```python
from build123d import *

# Parameters (mm, degrees)
SKETCH2_W           = 54
SKETCH2_H           = 6.2
BOSS_EXTRUDE2_DEPTH = 12.5
SKETCH3_R           = 2.8
CUT_EXTRUDE1_DEPTH  = 6.2
CUT_EXTRUDE2_DEPTH  = 1.9
SKETCH6_W           = 8.1
SKETCH6_H           = 4
CUT_EXTRUDE3_DEPTH  = 8.65741
SKETCH7_W           = 3
SKETCH7_H           = 25
BOSS_EXTRUDE3_DEPTH = 7.9
CUT_EXTRUDE4_DEPTH  = 2
SKETCH9_R           = 0.7
CUT_EXTRUDE5_DEPTH  = 2
SKETCH13_W          = 54
SKETCH13_H          = 2.82
CUT_EXTRUDE6_DEPTH  = 33.925066439
SKETCH18_W          = 3
SKETCH18_H          = 2.82
CUT_EXTRUDE9_DEPTH  = 10
SKETCH19_W          = 0.539072716
SKETCH19_H          = 14.1
CUT_EXTRUDE11_DEPTH = 57.508848865
CUT_EXTRUDE13_DEPTH = 2.5
CUT_EXTRUDE15_START = -2
SKETCH23_R          = 1.6
CUT_EXTRUDE15_DEPTH = 7
CUT_EXTRUDE16_DEPTH = 1.2
SKETCH26_W          = 5.64
SKETCH26_H          = 2.8
CUT_EXTRUDE17_DEPTH = 2.3
SKETCH29_W          = 9
SKETCH29_H          = 3
BOSS_EXTRUDE5_DEPTH = 7.9
SKETCH34_W          = 9
SKETCH34_H          = 7.9
BOSS_EXTRUDE6_DEPTH = 7.5
CUT_EXTRUDE19_DEPTH = 9
CUT_EXTRUDE20_DEPTH = 2.5
SKETCH31_R          = 1.5
CUT_EXTRUDE18_DEPTH = 37.30881069


with BuildPart() as part:
    # Sketch2 → Boss-Extrude2 (new, symmetric)
    with BuildSketch(Plane(origin=(10.528308017, 2.71655886, 0), x_dir=(1, 0, 0), z_dir=(0, 0, 1))):
        with Locations((-10.528308017, -2.71655886)):
            Rectangle(SKETCH2_W, SKETCH2_H)
    extrude(amount=BOSS_EXTRUDE2_DEPTH, both=True)

    # Sketch3 → Cut-Extrude1 (cut)
    with BuildSketch(Plane.XZ.offset(3.1)):
        with Locations((-12.165967216, -142.374755929)):
            Circle(SKETCH3_R)
    extrude(amount=-CUT_EXTRUDE1_DEPTH, mode=Mode.SUBTRACT)

    # Sketch4 → Cut-Extrude2 (cut, symmetric)
    with BuildSketch(Plane(origin=(0, 0, 0), x_dir=(1, 0, 0), z_dir=(0, 1, 0))):
        Polygon((-10.635076842, 0.660738766), (-14.535076842, 2.912404816), (-18.435076842, 0.660738766), (-18.435076842, -3.842593333), (-14.535076842, -6.094259383), (-10.635076842, -3.842593333), align=None)
    extrude(amount=CUT_EXTRUDE2_DEPTH, both=True, mode=Mode.SUBTRACT)

    # Sketch6 → Cut-Extrude3 (cut)
    with BuildSketch(Plane.XY.offset(12.5)):
        with Locations((-14.535076842, 0)):
            Rectangle(SKETCH6_W, SKETCH6_H)
    extrude(amount=-CUT_EXTRUDE3_DEPTH, mode=Mode.SUBTRACT)

    # Sketch7 → Boss-Extrude3 (add)
    with BuildSketch(Plane.XZ.offset(3.1)):
        with Locations((-25.5, 0)):
            Rectangle(SKETCH7_W, SKETCH7_H)
    boss_extrude3 = extrude(amount=BOSS_EXTRUDE3_DEPTH)

    # Sketch8 → Cut-Extrude4 (cut)
    with BuildSketch(Plane.ZY.offset(27)):
        with BuildLine():
            Line((-1.559072716, -7.9), (-1.559072716, -11))
            Line((-1.559072716, -11), (4.740927284, -11))
            Line((4.740927284, -11), (4.740927284, -7.9))
            ThreePointArc((4.740927284, -7.9), (1.590927284, -4.75), (-1.559072716, -7.9))
        make_face()
    cut_extrude4 = extrude(amount=-CUT_EXTRUDE4_DEPTH, mode=Mode.SUBTRACT)

    # Sketch9 → Cut-Extrude5 (cut)
    with BuildSketch(Plane(origin=(-24, 0, 0), x_dir=(0, 0, -1), z_dir=(1, 0, 0))):
        with Locations((142.374755929, -8.1)):
            Circle(SKETCH9_R)
    cut_extrude5 = extrude(amount=-CUT_EXTRUDE5_DEPTH, mode=Mode.SUBTRACT)

    # Sketch13 → Cut-Extrude6 (cut, through all)
    with BuildSketch(Plane(origin=(0, 3.1, 0), x_dir=(1, 0, 0), z_dir=(0, 1, 0))):
        with Locations((0, 11.09)):
            Rectangle(SKETCH13_W, SKETCH13_H)
    extrude(amount=-CUT_EXTRUDE6_DEPTH, mode=Mode.SUBTRACT)

    # Mirror1: Boss-Extrude3, Cut-Extrude4, Cut-Extrude5 across plane
    add(boss_extrude3.mirror(Plane.ZY.offset(14.535076842)))
    add(cut_extrude4.mirror(Plane.ZY.offset(14.535076842)), mode=Mode.SUBTRACT)
    add(cut_extrude5.mirror(Plane.ZY.offset(14.535076842)), mode=Mode.SUBTRACT)

    # Sketch18 → Cut-Extrude9 (cut)
    with BuildSketch(Plane(origin=(0, -3.1, 0), x_dir=(1, 0, 0), z_dir=(0, 1, 0))):
        with Locations((-3.570153685, 11.09)):
            Rectangle(SKETCH18_W, SKETCH18_H)
    extrude(amount=-CUT_EXTRUDE9_DEPTH, mode=Mode.SUBTRACT)

    # Sketch19 → Cut-Extrude11 (cut, through all)
    with BuildSketch(Plane.ZY.offset(27)):
        with Locations((12.230463642, -3.95)):
            Rectangle(SKETCH19_W, SKETCH19_H)
    extrude(amount=-CUT_EXTRUDE11_DEPTH, mode=Mode.SUBTRACT)

    # Sketch22 → Cut-Extrude13 (cut)
    with BuildSketch(Plane.XZ.offset(3.1)):
        Polygon((15, 10.472778345), (12.15, 8.827330078), (12.15, 5.536433544), (15, 3.890985277), (17.85, 5.536433544), (17.85, 8.827330078), align=None)
        Polygon((15, -2.584684642), (12.15, -4.230132909), (12.15, -7.521029443), (15, -9.16647771), (17.85, -7.521029443), (17.85, -4.230132909), align=None)
    extrude(amount=-CUT_EXTRUDE13_DEPTH, mode=Mode.SUBTRACT)

    # Sketch23 → Cut-Extrude15 (cut)
    with BuildSketch(Plane(origin=(0, 3.1, 0), x_dir=(1, 0, 0), z_dir=(0, 1, 0)).offset(CUT_EXTRUDE15_START)):
        with Locations((-0.270153685, 292.910439142)):
            Circle(SKETCH23_R)
        with Locations(Location((-0.270153685, -8.160927284, 0), (0, 0, 180))):
            Circle(SKETCH23_R)
    extrude(amount=-CUT_EXTRUDE15_DEPTH, mode=Mode.SUBTRACT)

    # Sketch24 → Cut-Extrude16 (cut, symmetric)
    with BuildSketch(Plane(origin=(0, 0, 0), x_dir=(1, 0, 0), z_dir=(0, 1, 0))):
        Polygon((-0.270153685, -11.451823818), (2.579846315, -9.806375551), (2.579846315, -6.515479016), (-0.270153685, -4.870030749), (-3.120153685, -6.515479016), (-3.120153685, -9.806375551), align=None)
        Polygon((-0.270153685, 1.688176182), (2.579846315, 3.333624449), (2.579846315, 6.624520984), (-0.270153685, 8.269969251), (-3.120153685, 6.624520984), (-3.120153685, 3.333624449), align=None)
    extrude(amount=CUT_EXTRUDE16_DEPTH, both=True, mode=Mode.SUBTRACT)

    # Sketch26 → Cut-Extrude17 (cut)
    with BuildSketch(Plane.XY.offset(11.960927284)):
        with Locations((0.08, 0)):
            Rectangle(SKETCH26_W, SKETCH26_H)
    cut_extrude17 = extrude(amount=-CUT_EXTRUDE17_DEPTH, mode=Mode.SUBTRACT)

    # Mirror4: Cut-Extrude17 across plane
    add(cut_extrude17.mirror(Plane(origin=(0, 0, 1.140463642), x_dir=(1, 0, 0), z_dir=(0, 0, -1))), mode=Mode.SUBTRACT)

    # Sketch29 → Boss-Extrude5 (add)
    with BuildSketch(Plane.XZ.offset(3.1)):
        with Locations((22.5, 10.460927284)):
            Rectangle(SKETCH29_W, SKETCH29_H)
        with Locations((-22.5, 10.460927284)):
            Rectangle(SKETCH29_W, SKETCH29_H)
    boss_extrude5 = extrude(amount=BOSS_EXTRUDE5_DEPTH)

    # Mirror5: Boss-Extrude5 across plane
    add(boss_extrude5.mirror(Plane(origin=(0, 0, 1.140463642), x_dir=(1, 0, 0), z_dir=(0, 0, -1))))

    # Sketch34 → Boss-Extrude6 (add, symmetric)
    with BuildSketch(Plane(origin=(0, 0, 1.140463642), x_dir=(-1, 0, 0), z_dir=(0, 0, -1))):
        with Locations((-22.5, -7.05)):
            Rectangle(SKETCH34_W, SKETCH34_H)
    extrude(amount=BOSS_EXTRUDE6_DEPTH, both=True)

    # Sketch35 → Cut-Extrude19 (cut)
    with BuildSketch(Plane(origin=(27, 0, 0), x_dir=(0, 0, -1), z_dir=(1, 0, 0))):
        with BuildLine():
            Line((-4.740927284, -11), (1.559072716, -11))
            Line((1.559072716, -11), (1.559072716, -7.9))
            ThreePointArc((1.559072716, -7.9), (-1.590927284, -4.75), (-4.740927284, -7.9))
            Line((-4.740927284, -7.9), (-4.740927284, -11))
        make_face()
    extrude(amount=-CUT_EXTRUDE19_DEPTH, mode=Mode.SUBTRACT)

    # Sketch36 → Cut-Extrude20 (cut)
    with BuildSketch(Plane.XZ.offset(11)):
        with BuildLine():
            Line((-18, -150.496582169), (-18, -147.496582169))
            Line((-18, -147.496582169), (-20.754732899, -147.496582169))
            ThreePointArc((-20.754732899, -147.496582169), (-19.531717613, -149.138314245), (-18, -150.496582169))
        make_face()
        with BuildLine():
            Line((-20.754732899, -137.252929689), (-18, -137.252929689))
            Line((-18, -137.252929689), (-18, -134.252929689))
            ThreePointArc((-18, -134.252929689), (-19.531717613, -135.611197614), (-20.754732899, -137.252929689))
        make_face()
    extrude(amount=-CUT_EXTRUDE20_DEPTH, mode=Mode.SUBTRACT)

    # Sketch31 → Cut-Extrude18 (cut, through all)
    with BuildSketch(Plane(origin=(0, 0, -9.68), x_dir=(-1, 0, 0), z_dir=(0, 0, -1))):
        with Locations(Location((-21.66, -5.4, 0), (0, 0, 90))):
            Circle(SKETCH31_R)
        with Locations((21.5, -5.4)):
            Circle(SKETCH31_R)
    extrude(amount=-CUT_EXTRUDE18_DEPTH, mode=Mode.SUBTRACT)


solid = part.part
```
Work out the finished part from the listing and answer in its coordinate system (mm). A direction names the side the tool comes from. Give positions to 0.01 mm unless a question says otherwise; leave off trailing zeros. Write each loop counter-clockwise with the first axis right and the second up, starting at its lowest first coordinate (ties: lowest second). Pieces come first, ordered by that corner, then holes. Notation, with made-up numbers: (4.5, 72.5) - (41.5, 72.5) arc R27 ccw to (41.5, 92.5) - close; hole circle Ø9 at (-37.75, 62). An arc over 180 degrees is marked (long way). Use one line per item in the form item = value.
1. For faces 1 (the face through (-15, -2, 8)), 2 (the face through (16.4, -1.9, 4.7)), 3 (the face through (22, -11, -8)), 4 (the face through (-3.06, -4.75, 1.66)), 5 (the face through (0, -1.2, -5)), determine the directions among +Z, -Z, +X, -X, +Y, -Y from which every point of the face is accessible in a straight line to the end or side of a thin tool.
Filled in:
face_1 = +Z
face_2 = -Y
face_3 = +Z, -Z, +X, -X, -Y
face_4 = +X, -Y
face_5 = none
2. A cutting plane is placed at C-C (y = -2.5). Write down the section's boundary in (x, z), and give its area (3 significant figures).
Filled in:
outline = (-27, -9.68) - (27, -9.68) - (27, 11.96) - (-27, 11.96) - close; hole circle Ø3.2 at (-0.27, 8.16); hole (12.15, -7.52) - (15, -9.17) - (17.85, -7.52) - (17.85, -4.23) - (15, -2.58) - (12.15, -4.23) - close; hole (12.15, 5.54) - (15, 3.89) - (17.85, 5.54) - (17.85, 8.83) - (15, 10.47) - (12.15, 8.83) - close
area = 1,100 mm^2
3. A cutting plane is placed at B-B (x = 16.5). Write down the section's boundary in (y, z), and give its area (3 significant figures).
Filled in:
outline = (-3.1, -9.68) - (3.1, -9.68) - (3.1, 11.96) - (-3.1, 11.96) - (-3.1, 9.61) - (-0.6, 9.61) - (-0.6, 4.76) - (-3.1, 4.76) - (-3.1, -3.45) - (-0.6, -3.45) - (-0.6, -8.3) - (-3.1, -8.3) - close
area = 110 mm^2
4. Each of these flat-tipped pins is pushed along its axis until it touches: pin 1 Ø1.7 at (x, z) = (15.5, -4.5) entering from -Y; pin 2 Ø1.9 at (y, z) = (-7, 2.5) entering from -X; pin 3 Ø5 at (x, z) = (1.5, 1) entering from -Y. Where does it stop, or does it pass through?
Filled in:
pin_1 = -0.6
pin_2 = -25
pin_3 = -3.1
5. Determine the mould class of faces 6 (the face through (23, -7, 8.64)), 7 (the face through (0, -2, 11.961)), 8 (the face through (-18, -7, 10)) for opening direction Z: released by +Z, released by -Z, zero draft, split by the parting line, or undercut.
Filled in:
face_6 = undercut
face_7 = released by +Z
face_8 = zero draft
6. A cutting plane is placed at A-A (z = -5.5). Write down the section's boundary in (x, y).
Filled in:
outline = (-27, -11) - (-24, -11) - (-24, -3.1) - (-5.07, -3.1) - (-5.07, -11) - (-2.07, -11) - (-2.07, -3.1) - (12.15, -3.1) - (12.15, -0.6) - (17.85, -0.6) - (17.85, -3.1) - (18, -3.1) - (18, -11) - (27, -11) - (27, 3.1) - (-27, 3.1) - close; hole (-3.12, -1.2) - (2.58, -1.2) - (2.58, 1.2) - (-3.12, 1.2) - close; hole circle Ø3 at (21.66, -5.4)
7. A cutting plane is placed at D-D (y = -10). State how many separate pieces and enclosed holes the cut face has, and give its area (3 significant figures).
Filled in:
separate_pieces = 6
enclosed_holes = 0
area = 273 mm^2
8. Consider L1, parallel to X at y = -3.5, z = 3.75; L2, parallel to X at y = -0.25, z = 10.25; L3, parallel to Z at x = 23, y = -9. Determine where each line is inside the solid, lowest interval first.
Filled in:
L1 = -27 to -24, -5.07 to -2.07, 18 to 27
L2 = -27 to -18.59, -10.49 to -2.74, 2.9 to 27
L3 = -9.68 to -6.68, -6.36 to -1.56, 4.74 to 8.64, 8.96 to 11.96
